Geometry: final body of the model. Coordinates: model frame, mm. A direction names the side the tool comes from. Give positions to 0.01 mm unless a question says otherwise; leave off trailing zeros. Write each loop counter-clockwise with the first axis right and the second up, starting at its lowest first coordinate (ties: lowest second). Pieces come first, ordered by that corner, then holes.
Q1. Reachability of faces 1 (the face through (-22, 38, -8)), 2 (the face through (-3.228, 8.792, 0.406)) from +Z, -Z, +X, -X, +Y, -Y: full face, straight path, thin tool, end or side. Return the list, or none.
Q2. Line query: L1, parallel to X at y = 5, z = 0.5; L2, parallel to X at y = 12.25, z = 0; L3, parallel to Y at x = -7.5, z = -1.5. Output: solid intervals per line, ascending.
Q3. Pin query (flat end, axial travel): pin 1 (14 mm diameter, centred on x = -21, y = 36.5, fed in from +Z); pin 2 (10 mm diameter, centred on x = -24.5, y = 32, fed in from -Z); pin 3 (1 mm diameter, centred on y = 18.5, z = -18.5, fed in from -X). Return the tip coordinate at first contact, or that it passes through.
Q4. Draft query along X for faces 3 (the face through (21, 20, 0)), 4 (the face through (24.47, 9.86, 0.46)), 5 (the face through (-15.144, 38, 0)), 6 (the face through (28.977, 29.58, 1.162)). Return one class per face: pulls with the +X half, pulls with the -X half, needs draft (parallel to the pull), parting line crosses it, or undercut.
Q5. Cut plane A-A on x = -21.5. Return the cut outline in (y, z).
Q6. Cut plane D-D on y = 14.5. Return the cut outline in (x, z).
Q7. Cut plane B-B on z = 0. Return the cut outline in (x, y).
Q8. Cut plane C-C on x = 21. Return the cut outline in (y, z), plus the area to 3 significant figures.
```python
from build123d import *

# Parameters (mm, degrees)
SKETCH5_R           = 29
BOSS_EXTRUDE2_DEPTH = 60
CUT_EXTRUDE1_DEPTH  = 58
CUT_EXTRUDE3_START  = -8
CUT_EXTRUDE3_DEPTH  = 16
SKETCH10_R          = 3.5
CUT_EXTRUDE4_DEPTH  = 20


# Read off the part's stored shape, not the designer's step: Cut-Extrude3
with BuildPart() as part:
    # Sketch5 → Boss-Extrude2 (new body)
    with BuildSketch(Plane(origin=(0, 0, 0), x_dir=(1, 0, 0), z_dir=(0, 1, 0))):
        with Locations(Location((0, 0, 0), (0, 0, 270))):
            Circle(SKETCH5_R)
    extrude(amount=BOSS_EXTRUDE2_DEPTH)

    # Sketch7 → Cut-Extrude1 (cut)
    with BuildSketch(Plane.XY.offset(29)):
        Polygon((12, 0), (-29, 23.671361037), (-29, 0), align=None)
    extrude(amount=-CUT_EXTRUDE1_DEPTH, mode=Mode.SUBTRACT)

    # Cut-Extrude3 outline → Cut-Extrude3 (cut)
    with BuildSketch(Plane.XY.offset(CUT_EXTRUDE3_START)):
        Polygon((-29, 23.671361037), (-15.143593539, 15.671361037), (-15.143593539, 60), (-30, 60), (-30, 24.248711306), align=None)
    extrude(amount=CUT_EXTRUDE3_DEPTH, mode=Mode.SUBTRACT)

    # Sketch10 → Cut-Extrude4 (cut)
    with BuildSketch(Plane.XZ):
        with Locations(Location((21, 0, 0), (0, 0, 270))):
            Circle(SKETCH10_R)
    extrude(amount=-CUT_EXTRUDE4_DEPTH, mode=Mode.SUBTRACT)


solid = part.part
```
Data:
1. face 1: -X, +Y, -Y
1. face 2: +Z, -Z, -X, -Y
2. L1: x = 3.34 to 17.54, 24.46 to 29
2. L2: x = -9.22 to 17.5, 24.5 to 29
2. L3: y = 11.26 to 60
3. pin 1: stops at z = 25.4
3. pin 2: stops at z = -21.47
3. pin 3: stops at x = -20.91
4. face 3: undercut
4. face 4: undercut
4. face 5: pulls with the -X half
4. face 6: parting line crosses it
5. outline: (19.34, -19.46) - (60, -19.46) - (60, -8) - (19.34, -8) - close; (19.34, 8) - (60, 8) - (60, 19.46) - (19.34, 19.46) - close
6. outline: (-13.11, -25.87) arc R29 ccw (long way) to (-13.11, 25.87) - close; hole circle Ø7 at (21, 0)
7. outline: (-15.14, 15.67) - (12, 0) - (17.5, 0) - (17.5, 20) - (24.5, 20) - (24.5, 0) - (29, 0) - (29, 60) - (-15.14, 60) - close
8. outline: (0, -20) - (60, -20) - (60, 20) - (0, 20) - (0, 3.5) - (20, 3.5) - (20, -3.5) - (0, -3.5) - close
8. area: 2,260 mm2
